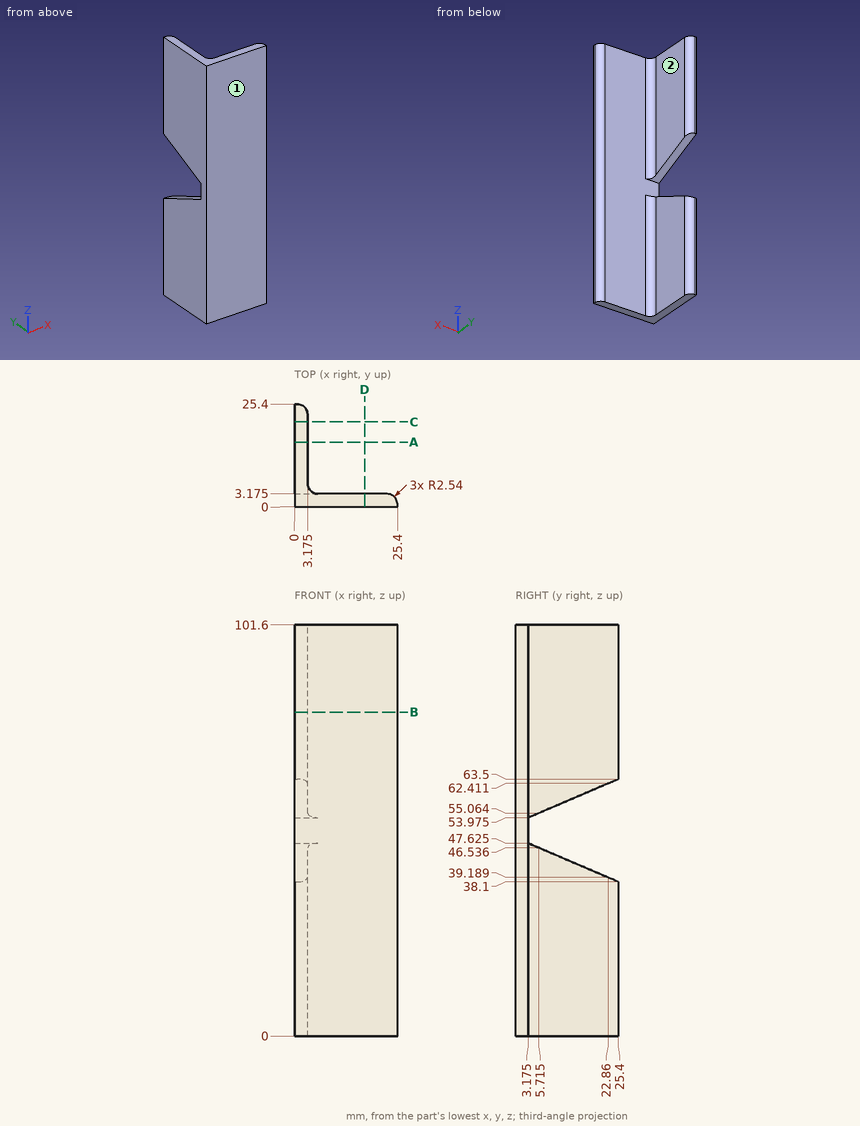
Part print with two shaded views. Sizes in mm from the minimum x, y, z corner. A direction names the side the tool comes from. Round coordinates to 2 decimals unless told otherwise and drop trailing zeros. Order: outer loops, then holes, each group sorted by start corner. A loop starts at its lowest first (then second) coordinate and runs counter-clockwise, first axis right, second up. Notation, with made-up numbers: (48.25, 87) -> (77.25, 87) arc R28 ccw to (77.25, 121) -> close; hole circle Ø10 at (72.5, 54). An arc over 180 degrees is marked (long way). Write each question's results on one line, items separated by ' | '.
1. Cut at A-A (y = 16). Give the cut face in (x, z) (1 decimal).
Findings below:
outline: (0, 0) -> (3.2, 0) -> (3.2, 42.1) -> (0, 42.1) -> close; (0, 59.5) -> (3.2, 59.5) -> (3.2, 101.6) -> (0, 101.6) -> close
2. 3-axis set-ups, long thin cutter, end or side, ignore diameter. For the marked faces 1 and 2: which of +Z, -Z, +X, -X, +Y, -Y reach the whole face in a straight line?
Findings below:
face 1: +Z, -Z, +X, -X, -Y | face 2: +Z, -Z, +X, +Y
3. Wall check: line 1 along X through (y, z) = (21, 83.5) (1 decimal); line 2 along X through (y, z) = (3.5, 61) (1 decimal). Give the ranges that are in metal, low to high. Write a range as [from, to].
Findings below:
line 1: x = [0, 3.2] | line 2: x = [0, 4.5]
4. Cut at B-B (z = 80). Give the cut face in (x, y) (1 decimal).
Findings below:
outline: (0, 0) -> (25.4, 0) -> (25.4, 0.6) arc R2.5 ccw to (22.9, 3.2) -> (5.7, 3.2) arc R2.5 cw to (3.2, 5.7) -> (3.2, 22.9) arc R2.5 ccw to (0.6, 25.4) -> (0, 25.4) -> close
5. Cut at C-C (y = 21). Give the cut face in (x, z) (1 decimal).
Findings below:
outline: (0, 0) -> (3.2, 0) -> (3.2, 40) -> (0, 40) -> close; (0, 61.6) -> (3.2, 61.6) -> (3.2, 101.6) -> (0, 101.6) -> close
6. Cut at D-D (x = 17.25). Give the cut face in (y, z) (1 decimal).
Findings below:
outline: (0, 0) -> (3.2, 0) -> (3.2, 101.6) -> (0, 101.6) -> close
7. Flat gauge pins, fed straight in: P1, Ø6, axis at x = 6.5, y = 9, coming from the +Z side; P2, Ø5, axis at x = 12.5, z = 46.5, coming from the +Y side (3 decimals); P3, Ø6, axis at y = 11.5, z = 37.5, coming from the +X side (3 decimals). Where does each tip first touch, or does it go through?
Findings below:
P1: passes through | P2: stops at y = 3.175 | P3: stops at x = 3.175
